Model file for the job. Use its own axes, mm. A direction names the side the tool comes from. Coordinates: 2 decimals unless noted, no trailing zeros. Loops run counter-clockwise (first coordinate to the right, second up) from the corner with the lowest first, then second, coordinate; pieces in that order, holes last.
from build123d import *

# Parameters (mm, degrees)
SKETCH1_W                  = 152.4
SKETCH1_H                  = 152.4
EXTRUDE1_DEPTH             = 6.35
SKETCH3_OUTSIDE_W          = 197.524
SKETCH3_OUTSIDE_H          = 197.524
EXTRUDE3_DEPTH             = 108.95
F_10_24_TAPPED_HOLE2_D     = 3.7973
F_10_24_TAPPED_HOLE2_DEPTH = 14.986
F_10_24_TAPPED_HOLE2_TIP   = 1.140824014
EXTRUDE4_DEPTH             = 3.175
SKETCH20_W                 = 12.7
SKETCH20_H                 = 25.4
EXTRUDE5_DEPTH             = 3.175


with BuildPart() as part:
    # Sketch1 → Extrude1 (new body)
    with BuildSketch(Plane.XY):
        Rectangle(SKETCH1_W, SKETCH1_H)
    extrude(amount=EXTRUDE1_DEPTH)

    # Sketch3 outside → Extrude3 (cut, through all)
    with BuildSketch(Plane.XY.offset(6.35)):
        Rectangle(SKETCH3_OUTSIDE_W, SKETCH3_OUTSIDE_H)
        Polygon((57.15, 76.2), (57.15, 12.7), (76.2, 12.7), (76.2, -12.7), (57.15, -12.7), (57.15, -76.2), (31.75, -76.2), (31.75, -12.7), (-76.2, -12.7), (-76.2, 12.7), (31.75, 12.7), (31.75, 76.2), align=None, mode=Mode.SUBTRACT)
    extrude(amount=-EXTRUDE3_DEPTH, mode=Mode.SUBTRACT)

    # Sketch11 → CSK for 1/4 Flat Head Socket Cap Screw2 (revolve, cut)
    with BuildSketch(Plane(origin=(-21.16074, -8.054e-06, 0), x_dir=(0, 1, 0), z_dir=(1, 0, 0))):
        Polygon((0, 0), (0, 6.35), (3.3782, 6.35), (3.3782, 3.728390023), (6.61924, 0), align=None)
    revolve(axis=Axis((-21.16074, -8.054e-06, -6.35), (0, 0, 1)), mode=Mode.SUBTRACT)

    # Sketch13 → CSK for 1/4 Flat Head Socket Cap Screw3 (revolve, cut)
    with BuildSketch(Plane(origin=(44.45, -8.054e-06, 0), x_dir=(0, 1, 0), z_dir=(1, 0, 0))):
        Polygon((0, 0), (0, 6.35), (3.3782, 6.35), (3.3782, 3.728390023), (6.61924, 0), align=None)
    revolve(axis=Axis((44.45, -8.054e-06, -6.35), (0, 0, 1)), mode=Mode.SUBTRACT)

    # #10-24 Tapped Hole2
    with Locations(Plane(origin=(-63.5, 0, 0), x_dir=(-1, 0, 0), z_dir=(0, 0, -1))):
        with Locations((0, 0), (-107.95, 62.23), (-107.95, -62.23)):
            Hole(F_10_24_TAPPED_HOLE2_D / 2, depth=F_10_24_TAPPED_HOLE2_DEPTH)
            with Locations((0, 0, -(F_10_24_TAPPED_HOLE2_DEPTH + F_10_24_TAPPED_HOLE2_TIP / 2))):  # 118° drill point
                Cone(0, F_10_24_TAPPED_HOLE2_D / 2, F_10_24_TAPPED_HOLE2_TIP, mode=Mode.SUBTRACT)

    # Sketch18 → Extrude4 (cut)
    with BuildSketch(Plane.XY.offset(6.35)):
        Polygon((-27.51074, 12.7), (-27.51074, -12.702586498), (-14.81074, -12.7), (-14.81074, 12.7), align=None)
    extrude(amount=-EXTRUDE4_DEPTH, mode=Mode.SUBTRACT)

    # Sketch20 → Extrude5 (cut)
    with BuildSketch(Plane.XY.offset(6.35)):
        with Locations((44.45, 0)):
            Rectangle(SKETCH20_W, SKETCH20_H)
    extrude(amount=-EXTRUDE5_DEPTH, mode=Mode.SUBTRACT)


solid = part.part
Q1. Drill centre lines: line 1 (Y direction, x = 44.45, z = 3.75); line 2 (Y direction, x = 44.45, z = 2.25); line 3 (X direction, y = 3, z = 1.5). Where is each one in solid material? Low to high.
Answers:
line 1: y = -76.2 to -64.13, -60.33 to -12.7, 12.7 to 60.33, 64.13 to 76.2
line 2: y = -76.2 to -64.13, -60.33 to -4.66, 4.66 to 60.33, 64.13 to 76.2
line 3: x = -76.2 to -25.55, -16.77 to 40.06, 48.84 to 76.2
Q2. Slice it at A-A (z = 4.75). List the corners of the cut face in (x, y), and give its area (3 significant figures).
Answers:
outline: (-76.2, -12.7) - (-27.51, -12.7) - (-27.51, 12.7) - (-76.2, 12.7) - close; (-14.81, -12.7) - (31.75, -12.7) - (31.75, -76.2) - (57.15, -76.2) - (57.15, -12.7) - (76.2, -12.7) - (76.2, 12.7) - (57.15, 12.7) - (57.15, 76.2) - (31.75, 76.2) - (31.75, 12.7) - (-14.81, 12.7) - close; hole circle Ø3.8 at (-63.5, 0); hole (38.1, -12.7) - (50.8, -12.7) - (50.8, 12.7) - (38.1, 12.7) - close; hole circle Ø3.8 at (44.45, -62.23); hole circle Ø3.8 at (44.45, 62.23)
area: 6,420 mm2
Q3. Which spindle directions (+Z, -Z, +X, -X, +Y, -Y) get a long thin tool onto all of the face, cutting with end or side? Do faces 1 (the flat face through (31.75, -45, 3)), 2 (the flat face through (57.15, 45, 3)), 3 (the flat face through (41.5, 3, 3.175)), 4 (the flat face through (-23, 12.7, 3)), 5 (the flat face through (67, -12.7, 3)). Say none if no direction does.
Answers:
face 1: +Z, -Z, -X, -Y
face 2: +Z, -Z, +X, +Y
face 3: +Z
face 4: +Z, -Z, -X, +Y
face 5: +Z, -Z, +X, -Y
Q4. Slice it at C-C (x = -63.5). List the corners of the cut face in (y, z), and give its area (3 significant figures).
Answers:
outline: (-12.7, 0) - (-1.9, 0) - (-1.9, 6.35) - (-12.7, 6.35) - close; (1.9, 0) - (12.7, 0) - (12.7, 6.35) - (1.9, 6.35) - close
area: 137 mm2
Q5. Mould opens along X. For faces 6 (the flat face through (-24, 3, 3.175)), 7 (the flat face through (44, -76.2, 3)), 8 (the flat face through (57.15, -44, 3)) say: +X half, -X half, draft (parallel to the pull), parting line (faces both ways), or undercut.
Answers:
face 6: undercut
face 7: draft
face 8: +X half
Q6. Slice it at D-D (x = 44.45). List the corners of the cut face in (y, z) (3 decimals).
Answers:
outline: (-76.2, 0) - (-64.129, 0) - (-64.129, 6.35) - (-76.2, 6.35) - close; (-60.331, 0) - (-6.619, 0) - (-3.859, 3.175) - (-12.7, 3.175) - (-12.7, 6.35) - (-60.331, 6.35) - close; (3.859, 3.175) - (6.619, 0) - (60.331, 0) - (60.331, 6.35) - (12.7, 6.35) - (12.7, 3.175) - close; (64.129, 0) - (76.2, 0) - (76.2, 6.35) - (64.129, 6.35) - close
Q7. Slice it at B-B (y = -62.23). List the corners of the cut face in (x, z).
Answers:
outline: (31.75, 0) - (42.55, 0) - (42.55, 6.35) - (31.75, 6.35) - close; (46.35, 0) - (57.15, 0) - (57.15, 6.35) - (46.35, 6.35) - close
Q8. Flat gauge pins, fed straight in: P1, Ø4, axis at x = 46.5, y = 3.5, coming from the +Z side (3 decimals); P2, Ø3, axis at y = 45.5, z = 2.5, coming from the +X side; P3, Ø3, axis at x = -46, z = 4.5, coming from the -Y side; P4, Ø1, axis at x = 59, y = -61, coming from the +Z side. Where does each tip first touch, or does it go through?
Answers:
P1: stops at z = 3.175
P2: stops at x = 57.15
P3: stops at y = -12.7
P4: passes through
